Verification items for the finished model (mm, model axes). Face numbers are marked on the shaded views. A direction names the side the tool comes from. Coordinates: 2 decimals unless noted, no trailing zeros. Loops run counter-clockwise (first coordinate to the right, second up) from the corner with the lowest first, then second, coordinate; pieces in that order, holes last. Notation, with made-up numbers: (41, 3.25) -> (75, 3.25) arc R14 cw to (75, 29.25) -> close; hole circle Ø5 at (50, -31.5). An arc over 180 degrees is marked (long way). Answer as a JSON object with one key per item and string values. Group by question number.
Q1. Gauge pin test, flat ends, axial feed: pin 1 Ø0.6 at (x, y) = (-0.5, -1.5) entering from +Z; pin 2 Ø1.7 at (x, y) = (1.5, 6.5) entering from +Z; pin 3 Ø4 at (x, y) = (-2.5, -1) entering from -Z. Record the tip position at first contact, or that the pin passes through.
Q2. Cross-section at D-D on z = 30. Record the boundary of the cut face in (x, y), and give its area (3 significant figures).
Q3. Scan lines: L1, parallel to Y at x = -6, z = -24; L2, parallel to Z at x = -0.5, y = 1; L3, parallel to Z at x = 4.5, y = 1.5. Record each from-to range of solid material in increasing order.
Q4. Cross-section at C-C on z = 43. Record the boundary of the cut face in (x, y).
Q5. Set-up check for the marked faces 1, 2 and 3: record each of +Z, -Z, +X, -X, +Y, -Y from which the full face is reachable in a straight line by a thin tool's end or side.
Q6. Cross-section at A-A on x = 0. Record the boundary of the cut face in (y, z).
Q7. Cross-section at B-B on y = 1.25. Record the boundary of the cut face in (x, z), and give its area (3 significant figures).
```python
from build123d import *

# Parameters (mm, degrees)
SKETCH1_W           = 13.4
SKETCH1_H           = 123.3
BOSS_EXTRUDE1_DEPTH = 5.72
BOSS_EXTRUDE2_DEPTH = 13.4
BOSS_EXTRUDE3_DEPTH = 13.4
SKETCH5_W           = 8.5
SKETCH5_H           = 8.6
CUT_EXTRUDE1_DEPTH  = 13.4
BOSS_EXTRUDE4_DEPTH = 11.95
BOSS_EXTRUDE5_DEPTH = 11.95
CUT_EXTRUDE3_DEPTH  = 16.5
BOSS_EXTRUDE6_DEPTH = 11.95
CUT_EXTRUDE6_DEPTH  = 16.6
CUT_EXTRUDE7_DEPTH  = 16.6
BOSS_EXTRUDE7_DEPTH = 11.95
CUT_EXTRUDE8_DEPTH  = 16.6


with BuildPart() as part:
    # Sketch1 → Boss-Extrude1 (new body)
    with BuildSketch(Plane(origin=(0, 0, 0), x_dir=(1, 0, 0), z_dir=(0, 1, 0))):
        Rectangle(SKETCH1_W, SKETCH1_H)
        with BuildLine():
            ThreePointArc((-6.7, 61.65), (0, 68.35), (6.7, 61.65))
            Line((6.7, 61.65), (-6.7, 61.65))
        make_face()
    extrude(amount=BOSS_EXTRUDE1_DEPTH)

    # Sketch3 → Boss-Extrude2 (add)
    with BuildSketch(Plane(origin=(6.7, 0, 0), x_dir=(0, 0, -1), z_dir=(1, 0, 0))):
        Polygon((-49.73, 7.81), (-49.73, 5.72), (-33.53, 5.72), (-38.53, 7.81), align=None)
    extrude(amount=-BOSS_EXTRUDE2_DEPTH)

    # Sketch4 → Boss-Extrude3 (add)
    with BuildSketch(Plane(origin=(6.7, 0, 0), x_dir=(0, 0, -1), z_dir=(1, 0, 0))):
        Polygon((-49.73, 0), (-33.53, 0), (-38.53, -2.09), (-49.73, -2.09), align=None)
    extrude(amount=-BOSS_EXTRUDE3_DEPTH)

    # Sketch5 → Cut-Extrude1 (cut)
    with BuildSketch(Plane.XZ):
        with Locations((0, 57.35)):
            Rectangle(SKETCH5_W, SKETCH5_H)
    extrude(amount=-CUT_EXTRUDE1_DEPTH, mode=Mode.SUBTRACT)

    # Sketch6 → Boss-Extrude4 (add)
    with BuildSketch(Plane.XY.offset(61.65)):
        Polygon((-4.25, 5.72), (-6.7, 5.72), (-4.25, 7.81), align=None)
    extrude(amount=-BOSS_EXTRUDE4_DEPTH)

    # Sketch8 → Boss-Extrude5 (add)
    with BuildSketch(Plane.XY.offset(61.65)):
        Polygon((6.7, 5.72), (4.169608926, 7.81), (4.25, 5.72), align=None)
    extrude(amount=-BOSS_EXTRUDE5_DEPTH)

    # Sketch10 → Cut-Extrude3 (cut)
    with BuildSketch(Plane.XY.offset(49.73)):
        Polygon((-6.7, 7.81), (-6.7, 5.72), (-4.25, 7.81), align=None)
    extrude(amount=-CUT_EXTRUDE3_DEPTH, mode=Mode.SUBTRACT)

    # Sketch11 → Boss-Extrude6 (add)
    with BuildSketch(Plane.XY.offset(61.65)):
        Polygon((4.245506051, 0), (4.245506051, -2.09), (6.7, 0), align=None)
    extrude(amount=-BOSS_EXTRUDE6_DEPTH)

    # Sketch13 → Cut-Extrude6 (cut)
    with BuildSketch(Plane.XY.offset(49.73)):
        Polygon((6.7, 0), (4.245506051, -2.09), (6.7, -2.09), align=None)
    extrude(amount=-CUT_EXTRUDE6_DEPTH, mode=Mode.SUBTRACT)

    # Sketch14 → Cut-Extrude7 (cut)
    with BuildSketch(Plane.XY.offset(49.73)):
        Polygon((4.169608926, 7.81), (6.7, 7.81), (6.7, 5.72), align=None)
    extrude(amount=-CUT_EXTRUDE7_DEPTH, mode=Mode.SUBTRACT)

    # Sketch15 → Boss-Extrude7 (add)
    with BuildSketch(Plane.XY.offset(61.65)):
        Polygon((-4.25, -2.09), (-6.7, 0), (-4.25, 0), align=None)
    extrude(amount=-BOSS_EXTRUDE7_DEPTH)

    # Sketch16 → Cut-Extrude8 (cut)
    with BuildSketch(Plane.XY.offset(49.73)):
        Polygon((-6.7, 0), (-6.7, -2.09), (-4.25, -2.09), align=None)
    extrude(amount=-CUT_EXTRUDE8_DEPTH, mode=Mode.SUBTRACT)


solid = part.part
```
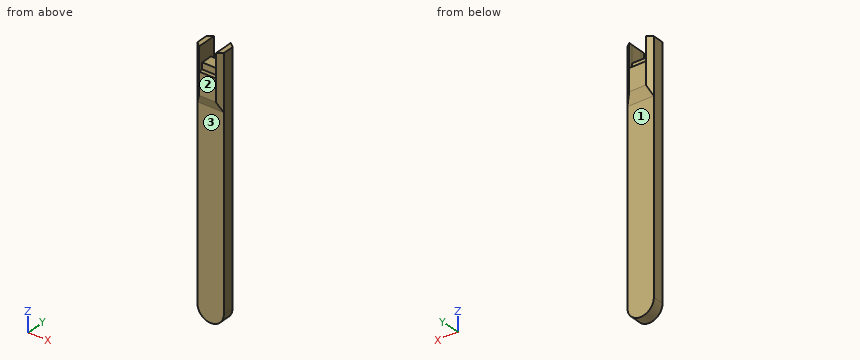
Computed values:
{
 "1": {"pin 1": "stops at z = 49.73", "pin 2": "stops at z = 53.05", "pin 3": "stops at z = -68.31"},
 "2": {"outline": "(-6.7, 0) -> (6.7, 0) -> (6.7, 5.72) -> (-6.7, 5.72) -> close", "area": "76.6 mm²"},
 "3": {"L1": "y = 0 to 5.72", "L2": "z = -68.33 to 53.05", "L3": "z = -66.61 to 61.65"},
 "4": {"outline": "(-6.7, 0) -> (-4.25, -2.09) -> (4.25, -2.09) -> (6.7, 0) -> (6.7, 5.72) -> (4.17, 7.81) -> (-4.25, 7.81) -> (-6.7, 5.72) -> close"},
 "5": {"face 1": "-Z, +X, -X, +Y", "face 2": "+Z, -Z, +X, -X, -Y", "face 3": "-Z, +X, -X, -Y"},
 "6": {"outline": "(-2.09, 38.53) -> (0, 33.53) -> (0, -68.35) -> (5.72, -68.35) -> (5.72, 33.53) -> (7.81, 38.53) -> (7.81, 49.73) -> (5.72, 49.73) -> (5.72, 53.05) -> (0, 53.05) -> (0, 49.73) -> (-2.09, 49.73) -> close"},
 "7": {"outline": "(-6.7, -61.65) arc R6.7 ccw to (6.7, -61.65) -> (6.7, 61.65) -> (4.25, 61.65) -> (4.25, 53.05) -> (-4.25, 53.05) -> (-4.25, 61.65) -> (-6.7, 61.65) -> close", "area": "1,650 mm²"}
}
